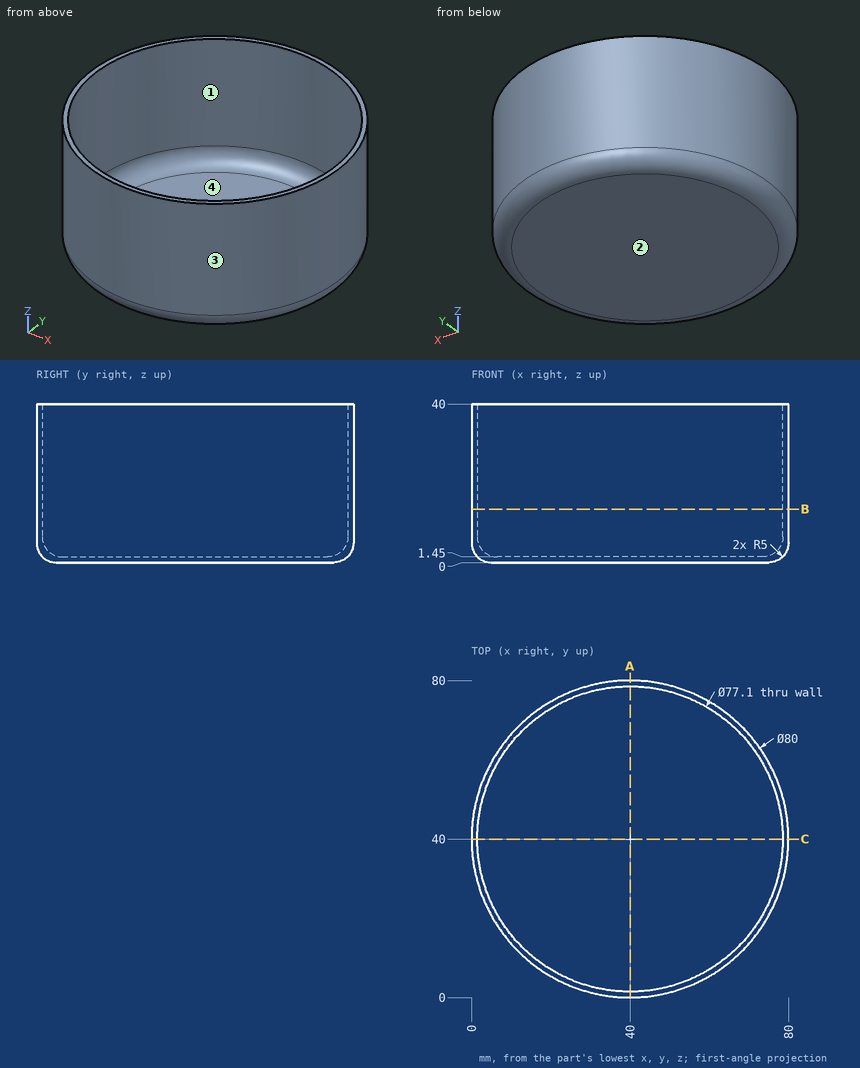
Could you check a few things on this drawing? It's one solid part, dimensions in mm from its lowest x, y, z. Give positions to 0.01 mm unless a question says otherwise; leave off trailing zeros. Loops run counter-clockwise (first coordinate to the right, second up) from the corner with the lowest first, then second, coordinate; pieces in that order, holes last. Notation, with made-up numbers: M 76,2 L 119,2 A23 cw 119,33 Z; hole C 67.25,19.25 d11. An arc over 180 degrees is marked long. One line per question, with ' | ' between items. Start each with the question number.
Q1. For pin 1 Ø5 at (x, z) = (66, 6) entering from -Y; pin 2 Ø4 at (x, z) = (14, 16) entering from +Y; pin 3 Ø5 at (y, z) = (27, 10) entering from -X, each with a flat end and sliding along its axis, tell me the tip position at first contact or that it passes through.
Q2. If I drill on line 1 (Y direction, x = 40, z = 24); line 2 (Z direction, x = 60.5, y = 43.5); line 3 (Y direction, x = 58.5, z = 13.5), over which ranges is the centre line in solid material (lowest first)? Write a range as from..to.
Q3. If we section it at B-B (z = 13.5): Please give me the cut outline in (x, y).
Q4. If we mould it in two halves opening along X, with no side actions, what happens to the marked faces 1, 2, 3 and 4? For each: +X half, -X half, draft (parallel to the pull), parting line (faces both ways), or undercut.
Q5. If we section it at A-A (x = 40): Please give me the cut outline in (y, z), plus the area to 3 significant figures.
Computed:
1) pin 1: stops at y = 7.63 | pin 2: stops at y = 72 | pin 3: stops at x = 1.4
2) line 1: y = 0..1.45, 78.55..80 | line 2: z = 0..1.45 | line 3: y = 4.54..6.18, 73.82..75.46
3) outline: C 40,40 d80; hole C 40,40 d77.1
4) face 1: undercut | face 2: draft | face 3: parting line | face 4: undercut
5) outline: M 0,5 A5 ccw 5,0 L 75,0 A5 ccw 80,5 L 80,40 L 78.55,40 L 78.55,6.45 A5 cw 73.55,1.45 L 6.45,1.45 A5 cw 1.45,6.45 L 1.45,40 L 0,40 Z | area: 228 mm²
